from build123d import *

# Parameters (mm, degrees)
SKETCH1_W                    = 99.06
SKETCH1_H                    = 73.66
BOSS_EXTRUDE1_DEPTH          = 25.4
M2_2X0_45_TAPPED_HOLE2_D     = 1.75
M2_2X0_45_TAPPED_HOLE2_DEPTH = 30.48
M2_2X0_45_TAPPED_HOLE2_TIP   = 0.525753042
SHELL3_T                     = -4.7625
FILLET2_R                    = 2.54
CUT_EXTRUDE1_DEPTH           = 109.694491581
CUT_EXTRUDE1_DEPTH_BACK      = 109.694491581
SKETCH11_R                   = 6
CUT_EXTRUDE2_DEPTH           = 93.326466953
CUT_EXTRUDE2_DEPTH_BACK      = 93.326466953
SKETCH12_W                   = 65.724340076
SKETCH12_H                   = 7.280106329


with BuildPart() as part:
    # Sketch1 → Boss-Extrude1 (new body)
    with BuildSketch(Plane(origin=(0, 0, 0), x_dir=(1, 0, 0), z_dir=(0, 1, 0))):
        Rectangle(SKETCH1_W, SKETCH1_H)
    extrude(amount=BOSS_EXTRUDE1_DEPTH)

    # M2.2x0.45 Tapped Hole2
    with Locations(Plane(origin=(0, 25.4, 0), x_dir=(1, 0, 0), z_dir=(0, 1, 0))):
        with Locations((-43.18, 30.48), (43.18, 30.48), (43.18, -30.48), (-43.18, -30.48)):
            Hole(M2_2X0_45_TAPPED_HOLE2_D / 2, depth=M2_2X0_45_TAPPED_HOLE2_DEPTH)
            with Locations((0, 0, -(M2_2X0_45_TAPPED_HOLE2_DEPTH + M2_2X0_45_TAPPED_HOLE2_TIP / 2))):  # 118° drill point
                Cone(0, M2_2X0_45_TAPPED_HOLE2_D / 2, M2_2X0_45_TAPPED_HOLE2_TIP, mode=Mode.SUBTRACT)

    # Shell3
    shell3_openings = [part.faces().sort_by_distance(p)[0] for p in [
        (0, 25.4, 0),
    ]]
    offset(amount=SHELL3_T, openings=shell3_openings, kind=Kind.INTERSECTION)

    # Fillet2
    fillet2_edges = [part.edges().sort_by_distance(p)[0] for p in [
        (-44.7675, 15.08125, -25.070633124),
        (-37.770633124, 15.08125, 32.0675),
        (44.7675, 15.08125, 25.070633124),
        (37.770633124, 15.08125, -32.0675),
        (-44.7675, 15.08125, 25.070633124),
        (37.770633124, 15.08125, 32.0675),
        (44.7675, 15.08125, -25.070633124),
        (-37.770633124, 15.08125, -32.0675),
    ]]
    fillet(fillet2_edges, radius=FILLET2_R)

    # Sketch11 → Cut-Extrude1 (cut, two sides: drawn at the far end of the back side and taken through both)
    with BuildSketch(Plane(origin=(49.53, 0, 0), x_dir=(0, 0, -1), z_dir=(1, 0, 0)).offset(-CUT_EXTRUDE1_DEPTH_BACK)):
        with Locations((-16.290648395, 12.7)):
            Circle(SKETCH11_R)
        with Locations((16.290648395, 12.7)):
            Circle(SKETCH11_R)
    extrude(amount=CUT_EXTRUDE1_DEPTH + CUT_EXTRUDE1_DEPTH_BACK, mode=Mode.SUBTRACT)

    # Sketch12 → Cut-Extrude2 (cut, two sides: drawn at the far end of the back side and taken through both)
    with BuildSketch(Plane(origin=(0, 0, -36.83), x_dir=(-1, 0, 0), z_dir=(0, 0, -1)).offset(-CUT_EXTRUDE2_DEPTH_BACK)):
        with Locations((-0.694647497, 12.759946836)):
            Rectangle(SKETCH12_W, SKETCH12_H)
    extrude(amount=CUT_EXTRUDE2_DEPTH + CUT_EXTRUDE2_DEPTH_BACK, mode=Mode.SUBTRACT)


solid = part.part
Build history of the part. All positions in model axes, mm. A direction names the side the tool comes from. Give positions to 0.01 mm unless a question says otherwise; leave off trailing zeros. Order: outer loops, then holes, each group sorted by start corner. A loop starts at its lowest first (then second) coordinate and runs counter-clockwise, first axis right, second up. Notation, with made-up numbers: M 85,74 L 112,74 A8 ccw 112,88 Z; hole C 40,14 d5. An arc over 180 degrees is marked long. Put each result on its own line as item: value.
Item 1: Probe line 1 (Z direction, x = -47, y = 12.7); line 2 (X direction, y = 7.5, z = -6); line 3 (Z direction, x = 19, y = 6.5). List the from-to ranges inside material, lowest first. Write a range as [from, to].
From the geometry:
line 1: z = [-36.83, -22.29], [-10.29, 10.29], [22.29, 36.83]
line 2: x = [-49.53, -44.77], [44.77, 49.53]
line 3: z = [-36.83, -32.07], [32.07, 36.83]
Item 2: Slice it at C-C, the plane y = 12.7. Give the number of separate pieces and of enclosed holes in the cut face, plus the area to 3 significant figures.
From the geometry:
separate pieces: 6
enclosed holes: 4
area: 882 mm2
Item 3: 3-axis set-ups, long thin cutter, end or side, ignore diameter. For faces 4 (the flat face through (0, 25.4, 33)), 5 (the cylindrical face through (44.14, 14.94, -24.03)), 6 (the flat face through (1, 9.12, 34)): which of +Z, -Z, +X, -X, +Y, -Y reach the whole face in a straight line?
From the geometry:
face 4: +Z, -Z, +X, -X, +Y
face 5: +Y
face 6: +Z, -Z
Item 4: Slice it at A-A, the plane x = -30. Write the cut outline in (y, z), plus the area to 3 significant figures.
From the geometry:
outline: M 0,-36.83 L 9.12,-36.83 L 9.12,-32.07 L 4.76,-32.07 L 4.76,32.07 L 9.12,32.07 L 9.12,36.83 L 0,36.83 Z; M 16.4,-36.83 L 25.4,-36.83 L 25.4,-32.07 L 16.4,-32.07 Z; M 16.4,32.07 L 25.4,32.07 L 25.4,36.83 L 16.4,36.83 Z
area: 478 mm2
Item 5: Flat gauge pins, fed straight in: pin 1 Ø6 at (x, z) = (3.5, -23) entering from -Y; pin 2 Ø9.5 at (y, z) = (12.7, 16.29) entering from -X; pin 3 Ø3 at (x, z) = (-5.5, -22.5) entering from +Y. Where does each tip first touch, or does it go through?
From the geometry:
pin 1: stops at y = 0
pin 2: passes through
pin 3: stops at y = 4.76
Item 6: Slice it at D-D, the plane z = -7. Write the cut outline in (x, y), plus the area to 3 significant figures.
From the geometry:
outline: M -49.53,0 L 49.53,0 L 49.53,25.4 L 44.77,25.4 L 44.77,4.76 L -44.77,4.76 L -44.77,25.4 L -49.53,25.4 Z
area: 668 mm2
Item 7: Two-plate mould, pull along X, no slides. Class faces 1 (the flat face through (-44.768, 15, 0)), 2 (the cylindrical face through (-47.2, 13, -10.3)), 3 (the flat face through (-49.53, 13, 1)): +X half, -X half, draft (parallel to the pull), parting line (faces both ways), or undercut.
From the geometry:
face 1: undercut
face 2: draft
face 3: -X half
Item 8: Slice it at B-B, the plane z = 14.5. Write the cut outline in (x, y).
From the geometry:
outline: M -49.53,0 L 49.53,0 L 49.53,6.97 L 44.77,6.97 L 44.77,4.76 L -44.77,4.76 L -44.77,6.97 L -49.53,6.97 Z; M -49.53,18.43 L -44.77,18.43 L -44.77,25.4 L -49.53,25.4 Z; M 44.77,18.43 L 49.53,18.43 L 49.53,25.4 L 44.77,25.4 Z
